```python
from build123d import *
from OCP.BRepAlgoAPI import BRepAlgoAPI_Cut
from OCP.TopTools import TopTools_ListOfShape

# Parameters (mm, degrees)
EXTRUDE_1_DEPTH          = 13.5
FILLET_1_R               = 0.5
CUT_EXTRUDE_1_DEPTH      = 2
CUT_EXTRUDE_1_DEPTH_BACK = 3.5
SKETCH_2_R               = 1
EXTRUDE_3_DEPTH          = 11.35
CUT_EXTRUDE_START        = -15.085786
SKETCH_14_W              = 17
SKETCH_14_H              = 6.5
CUT_EXTRUDE_7_DEPTH      = 15.085786
CUT_EXTRUDE_8_DEPTH      = 2
CUT_EXTRUDE_8_DEPTH_BACK = 15.5
SKETCH_15_R              = 1.150968548
SKETCH_15_R_2            = 1.118586154
FILLET_2_R               = 0.5
FILLET_START             = -5.25
FILLET_3_DEPTH           = 12.25
FILLET_START_2           = 3.25
FILLET_3_2_DEPTH         = 2
SKETCH_16_R              = 1.25
CUT_EXTRUDE_9_DEPTH      = 23.596980066
CHAMFER_2_SIZE           = 1.25


with BuildPart() as part:
    # 草图1 → 凸台-拉伸1 (new body)
    with BuildSketch(Plane(origin=(0, 0, 0), x_dir=(1, 0, 0), z_dir=(0, 1, 0))):
        Polygon((-5.5, -3.25), (-5.5, -5.25), (-10.5, -5.25), (-10.5, 5.25), (10.5, 5.25), (10.5, -5.25), (5.5, -5.25), (5.5, -3.25), (8.5, -3.25), (8.5, 3.25), (-8.5, 3.25), (-8.5, -3.25), align=None)
    extrude(amount=EXTRUDE_1_DEPTH)

    # 圆角1
    fillet_1_edges = [part.edges().sort_by_distance(p)[0] for p in [
        (-5.5, 6.75, 3.25),
        (-5.5, 6.75, 5.25),
        (-10.5, 6.75, 5.25),
        (10.5, 6.75, 5.25),
        (5.5, 6.75, 5.25),
        (5.5, 6.75, 3.25),
    ]]
    fillet(fillet_1_edges, radius=FILLET_1_R)

    # 草图2 → 切除-拉伸1 (cut, two sides: drawn at the far end of the back side and taken through both)
    with BuildSketch(Plane(origin=(0, 0, -5.25), x_dir=(-1, 0, 0), z_dir=(0, 0, -1)).offset(-CUT_EXTRUDE_1_DEPTH_BACK)):
        with Locations(Location((-6, 10.75, 0), (0, 0, 180))):
            Circle(SKETCH_2_R)
        with Locations(Location((6, 10.75, 0), (0, 0, 180))):
            Circle(SKETCH_2_R)
        with Locations(Location((6, 2.75, 0), (0, 0, 180))):
            Circle(SKETCH_2_R)
        with Locations(Location((-6, 2.75, 0), (0, 0, 180))):
            Circle(SKETCH_2_R)
    extrude(amount=CUT_EXTRUDE_1_DEPTH + CUT_EXTRUDE_1_DEPTH_BACK, mode=Mode.SUBTRACT)

    # 草图13 → 凸台-拉伸3 (add)
    with BuildSketch(Plane(origin=(0, 0, -5.25), x_dir=(-1, 0, 0), z_dir=(0, 0, -1))):
        with BuildLine():
            Line((7.999, -0.142846655), (7.999, 14.588591487))
            Line((7.999, 14.588591487), (10.999, 14.588591487))
            ThreePointArc((10.999, 14.588591487), (11.843623199, 14.420585487), (12.559660172, 13.942144877))
            ThreePointArc((12.559660172, 13.942144877), (12.884819299, 13.455509854), (12.999, 12.881484706))
            Line((12.999, 12.881484706), (12.999, -0.197194951))
            ThreePointArc((12.999, -0.197194951), (12.911132034, -0.409326985), (12.699, -0.497194951))
            Line((12.699, -0.497194951), (8.299, -0.497194951))
            ThreePointArc((8.299, -0.497194951), (8.075612065, -0.382152837), (7.999, -0.142846655))
        make_face()
    extrude(amount=-EXTRUDE_3_DEPTH)


with BuildPart() as cut_extrude_7_tool:
    # 草图14 → 切除-拉伸7 (new body)
    with BuildSketch(Plane.XZ.offset(0.497194951).offset(CUT_EXTRUDE_START)):
        Rectangle(SKETCH_14_W, SKETCH_14_H)
    extrude(amount=CUT_EXTRUDE_7_DEPTH)


with BuildPart() as part_1:
    add(part.part)

    # 切除-拉伸7: cut by cut_extrude_7_tool, with a tolerance
    cut_extrude_7_stock = TopTools_ListOfShape()
    cut_extrude_7_stock.Append(part_1.part.wrapped)
    cut_extrude_7_tools = TopTools_ListOfShape()
    cut_extrude_7_tools.Append(cut_extrude_7_tool.part.wrapped)
    cut_extrude_7_cut = BRepAlgoAPI_Cut()
    cut_extrude_7_cut.SetArguments(cut_extrude_7_stock)
    cut_extrude_7_cut.SetTools(cut_extrude_7_tools)
    cut_extrude_7_cut.SetFuzzyValue(0.00001)
    cut_extrude_7_cut.Build()
    add(Compound.cast(cut_extrude_7_cut.Shape()).solids(), mode=Mode.REPLACE)

    # 草图15 → 切除-拉伸8 (cut, two sides: drawn at the far end of the back side and taken through both)
    with BuildSketch(Plane.XY.offset(6.1).offset(-CUT_EXTRUDE_8_DEPTH_BACK)):
        with Locations(Location((-10.499, 12.002805049, 0), (0, 0, 180))):
            Circle(SKETCH_15_R)
        with Locations(Location((-10.499, 2.002805049, 0), (0, 0, 180))):
            Circle(SKETCH_15_R_2)
    extrude(amount=CUT_EXTRUDE_8_DEPTH + CUT_EXTRUDE_8_DEPTH_BACK, mode=Mode.SUBTRACT)

    # 圆角2
    fillet_2_edges = [part_1.edges().sort_by_distance(p)[0] for p in [
        (-7.999, 14.588591487, -4.25),
        (-7.999, 13.5, -4.25),
        (-7.999, 0, -4.25),
    ]]
    fillet(fillet_2_edges, radius=FILLET_2_R)

    # 圆角3: read off the stored shape, not the designer's step
    # 圆角3 outline → 圆角3 (cut)
    with BuildSketch(Plane.XY.offset(FILLET_START)):
        with BuildLine():
            Line((-7.999, 14.588591487), (-8.499, 14.588591487))
            ThreePointArc((-8.499, 14.588591487), (-8.14544661, 14.442144878), (-7.999, 14.088591487))
            Line((-7.999, 14.088591487), (-7.999, 14.588591487))
        make_face()
    extrude(amount=FILLET_3_DEPTH, mode=Mode.SUBTRACT)

    # Fillet 3 2 outline → Fillet 3 2 (add)
    with BuildSketch(Plane.XY.offset(FILLET_START_2)):
        with BuildLine():
            Line((-7.566440116, 0), (-7.999, 0))
            Line((-7.999, 0), (-7.999, -0.142846655))
            ThreePointArc((-7.999, -0.142846655), (-8.00224868, -0.223440354), (-8.025050148, -0.300809542))
            ThreePointArc((-8.025050148, -0.300809542), (-7.840670649, -0.081911954), (-7.566440116, 0))
        make_face()
        with BuildLine():
            ThreePointArc((-7.499, 13.5), (-7.852553391, 13.646446609), (-7.999, 14))
            Line((-7.999, 14), (-7.999, 13.5))
            Line((-7.999, 13.5), (-7.499, 13.5))
        make_face()
    extrude(amount=FILLET_3_2_DEPTH)

    # 草图16 → 切除-拉伸9 (cut, through all)
    with BuildSketch(Plane(origin=(0, 0, -5.25), x_dir=(-1, 0, 0), z_dir=(0, 0, -1))):
        with Locations((10.499, 12.002805049)):
            Circle(SKETCH_16_R)
        with Locations((10.499, 2.002805049)):
            Circle(SKETCH_16_R)
    extrude(amount=-CUT_EXTRUDE_9_DEPTH, mode=Mode.SUBTRACT)

    # 倒角2
    chamfer_2_edges = [part_1.edges().sort_by_distance(p)[0] for p in [
        (-9.249, 12.002805049, -5.25),
        (-9.249, 2.002805049, -5.25),
    ]]
    chamfer(chamfer_2_edges, length=CHAMFER_2_SIZE - 0.0001)  # a hair under: the kernel refuses the full size


solid = part_1.part
```
Can you work these out from the model? Positions are in its coordinate system, mm. A direction names the side the tool comes from. Round coordinates to 2 decimals unless told otherwise and drop trailing zeros. Loops run counter-clockwise (first coordinate to the right, second up) from the corner with the lowest first, then second, coordinate; pieces in that order, holes last.
Item 1: Suppose I cut it at D-D, the plane z = 5. Write out the boundary of the cut face in (x, y).
Item 2: Suppose I cut it at C-C, the plane y = 8. Write out the boundary of the cut face in (x, z), then the cut area to 3 significant figures.
Item 3: Will these pins go through, and if not, where does the flat tip stop? pin 1 Ø3 at (x, y) = (-6, 2.75) entering from -Z; pin 2 Ø4 at (x, z) = (6, 1.5) entering from -Y; pin 3 Ø2.5 at (x, y) = (6, 2.75) entering from +Z; pin 4 Ø1 at (x, z) = (-6.5, 4) entering from +Y.
Item 4: Please list where these lines run through material, in increasing order: L1, parallel to Y at x = -6, z = -3.9; L2, parallel to Z at x = -7.5, y = 10.75; L3, parallel to X at y = 3, z = -2.5.
Item 5: Suppose I cut it at A-A, the plane z = -0.75. Write out the boundary of the cut face in (x, y).
Item 6: Suppose I cut it at B-B, the plane x = 6.5. Write out the boundary of the cut face in (y, z).
Item 7: Which directions (+Z, -Z, +X, -X, +Y, -Y) give clear straight access to the entire face, cutting with the end or side of a thin tool? Please do faces 4 (the flat face through (-5.5, 7, 4)), 5 (the flat face through (4, 13.5, -4)), 6 (the cylindrical face through (-6.79, 3.36, -4.24)), 7 (the flat face through (7, 7, 3.25)).
Item 8: If we mould it in two halves opening along Z, with no side actions, what happens to faces 1 (the flat face through (-11, 7, 6.1)), 2 (the cylindrical face through (5.87, 9.76, -4.24)), 3 (the flat face through (8.5, 7, 0))? For each: +Z half, -Z half, draft (parallel to the pull), parting line (faces both ways), or undercut.
Reported:
1. outline: (-13, -0.2) arc R0.3 ccw to (-12.7, -0.5) - (-8.3, -0.5) arc R0.33 ccw to (-8.03, -0.3) arc R0.5 cw to (-7.57, 0) - (-5.57, 0) - (-5.57, 13.5) - (-7.5, 13.5) arc R0.5 cw to (-8, 14) - (-8, 14.09) arc R0.5 ccw to (-8.5, 14.59) - (-11, 14.59) arc R2.21 ccw to (-12.56, 13.94) arc R1.5 ccw to (-13, 12.88) - close; (5.57, 0) - (10.43, 0) - (10.43, 13.5) - (5.57, 13.5) - close; hole circle Ø2.5 at (-10.5, 2); hole circle Ø2.5 at (-10.5, 12)
2. outline: (-13, -5.25) - (10.5, -5.25) - (10.5, 4.75) arc R0.5 ccw to (10, 5.25) - (6, 5.25) arc R0.5 ccw to (5.5, 4.75) - (5.5, 3.75) arc R0.5 ccw to (6, 3.25) - (8.5, 3.25) - (8.5, -3.25) - (-8.5, -3.25) - (-8.5, 3.25) - (-6, 3.25) arc R0.5 ccw to (-5.5, 3.75) - (-5.5, 4.75) arc R0.5 ccw to (-6, 5.25) - (-8, 5.25) - (-8, 6.1) - (-13, 6.1) - close
2. area: 118 mm2
3. pin 1: stops at z = -5.25
3. pin 2: stops at y = 0
3. pin 3: stops at z = 5.25
3. pin 4: stops at y = 13.5
4. L1: y = 0 to 1.75, 3.75 to 9.75, 11.75 to 13.5
4. L2: z = -5.25 to -3.25, 3.25 to 5.25
4. L3: x = -13 to -11.25, -9.75 to -8.5, 8.5 to 10.5
5. outline: (-13, -0.2) arc R0.3 ccw to (-12.7, -0.5) - (-8.5, -0.5) - (-8.5, 14.59) - (-11, 14.59) arc R2.21 ccw to (-12.56, 13.94) arc R1.5 ccw to (-13, 12.88) - close; (8.5, 0) - (10.5, 0) - (10.5, 13.5) - (8.5, 13.5) - close; hole circle Ø2.5 at (-10.5, 2); hole circle Ø2.5 at (-10.5, 12)
6. outline: (0, -5.25) - (1.88, -5.25) - (1.88, -3.25) - (0, -3.25) - close; (0, 3.25) - (13.5, 3.25) - (13.5, 5.25) - (0, 5.25) - close; (3.62, -5.25) - (9.88, -5.25) - (9.88, -3.25) - (3.62, -3.25) - close; (11.62, -5.25) - (13.5, -5.25) - (13.5, -3.25) - (11.62, -3.25) - close
7. face 4: +Z, +Y, -Y
7. face 5: +Z, -Z, +X, +Y
7. face 6: -Z
7. face 7: +Y, -Y
8. face 1: +Z half
8. face 2: draft
8. face 3: undercut
